Job drawing, mm, ordinate dimensions from the low corner. One solid piece. Give positions to 0.01 mm unless a question says otherwise; leave off trailing zeros. Write each loop counter-clockwise with the first axis right and the second up, starting at its lowest first coordinate (ties: lowest second). Pieces come first, ordered by that corner, then holes. Notation, with made-up numbers: (-31, 49) -> (-26, 49) arc R22 cw to (-26, 61) -> close; hole circle Ø3 at (82.25, -25). An arc over 180 degrees is marked (long way). Put each result on its own line as item: value. Start each with the question number.
Item 1: Drill centre lines: line 1 along Y through (x, z) = (5, 7); line 2 along Y through (x, z) = (4, 8.5); line 3 along X through (y, z) = (57.5, 4.75). Where is each one in solid material? Low to high.
Item 2: Slice it at A-A, the plane z = 2. List the corners of the cut face in (x, y), plus the area to 3 significant figures.
Item 3: Slice it at B-B, the plane y = 6.5. List the corners of the cut face in (x, z), plus the area to 3 significant figures.
Item 4: Slice it at C-C, the plane y = 148.5. List the corners of the cut face in (x, z).
Item 5: Flat gauge pins, fed straight in: pin 1 Ø4 at (y, z) = (97, 1.5) entering from -X; pin 2 Ø4 at (x, y) = (8, 112.5) entering from -Z. Where does each tip first touch, or does it go through?
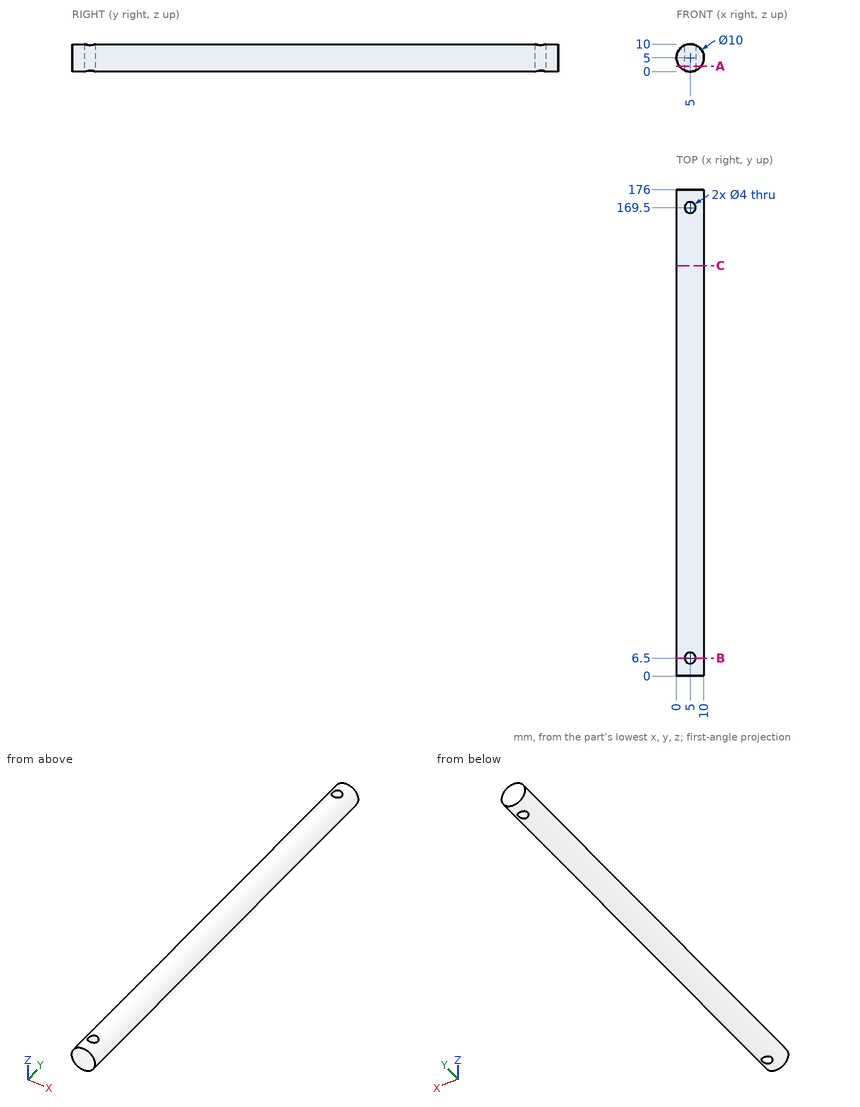
Values follow:
1. line 1: 0 to 4.5, 8.5 to 167.5, 171.5 to 176
1. line 2: 0 to 4.77, 8.23 to 167.77, 171.23 to 176
1. line 3: 0.01 to 9.99
2. outline: (1, 0) -> (9, 0) -> (9, 176) -> (1, 176) -> close; hole circle Ø4 at (5, 6.5); hole circle Ø4 at (5, 169.5)
2. area: 1,380 mm2
3. outline: (3, 0.42) -> (3, 9.58) arc R5 ccw to start; (7, 0.42) arc R5 ccw to (7, 9.58) -> close
3. area: 39.6 mm2
4. outline: circle Ø10 at (5, 5)
5. pin 1: x = 0.23
5. pin 2: z = 0.1
